For this review, use the dimensioned drawing (mm, ordinates from the lowest corner) and the shaded views. Coordinates: 2 decimals unless noted, no trailing zeros. Write each loop counter-clockwise with the first axis right and the second up, starting at its lowest first coordinate (ties: lowest second). Pieces come first, ordered by that corner, then holes.
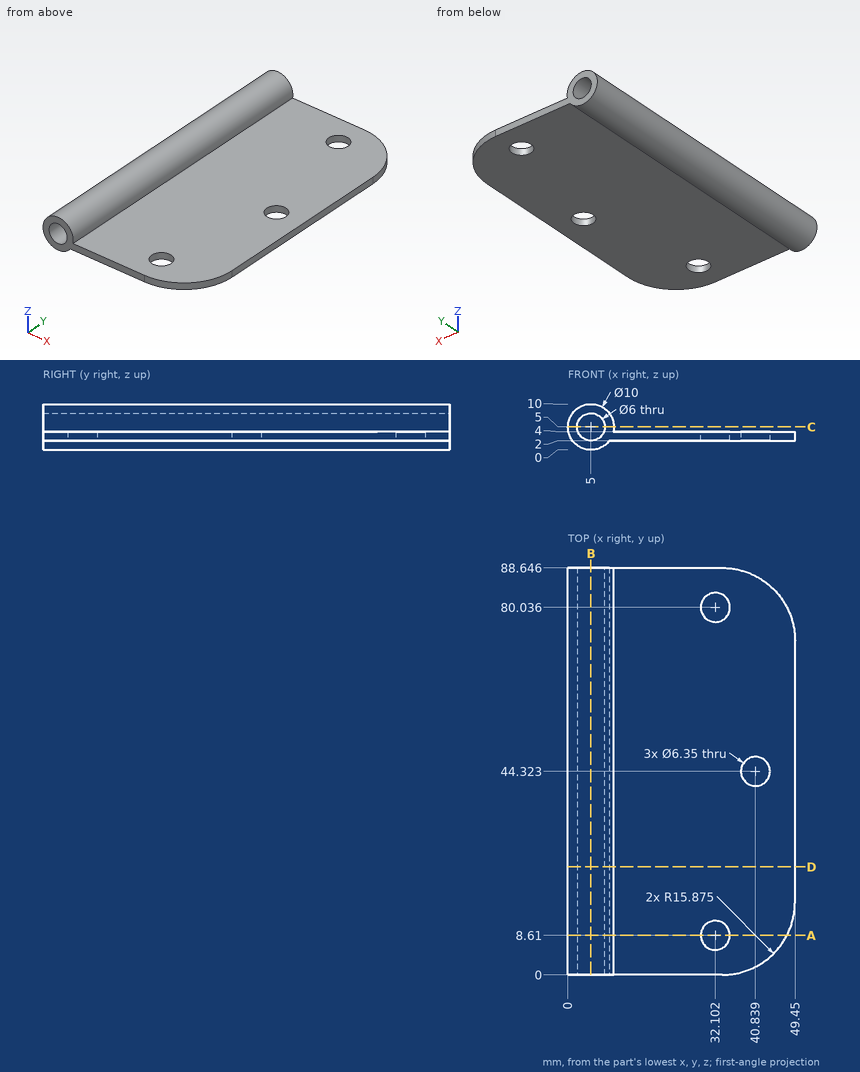
Item 1: Take a section at A-A, the plane y = 8.61. Write out the cut boundary in (x, z).
Solved:
outline: (9, 2) - (28.93, 2) - (28.93, 4) - (9.9, 4) arc R5 ccw (long way) to start; (35.28, 2) - (47.69, 2) - (47.69, 4) - (35.28, 4) - close; hole circle Ø6 at (5, 5)
Item 2: Take a section at D-D, the plane y = 23.5. Write out the cut boundary in (x, z).
Solved:
outline: (9, 2) - (49.45, 2) - (49.45, 4) - (9.9, 4) arc R5 ccw (long way) to start; hole circle Ø6 at (5, 5)
Item 3: For pin 1 (10 mm diameter, centred on x = 32.1, y = 80.04, fed in from +Z); pin 2 (5 mm diameter, centred on x = 17.5, y = 39, fed in from -Z); pin 3 (2 mm diameter, centred on x = 36, z = 4, fed in from -Y), all flat-tipped, find the tip position at first contact; note any pin that passes through.
Solved:
pin 1: stops at z = 4
pin 2: stops at z = 2
pin 3: stops at y = 0.06
Item 4: Take a section at C-C, the plane z = 5. Write out the cut boundary in (x, y).
Solved:
outline: (0, 0) - (2, 0) - (2, 88.65) - (0, 88.65) - close; (8, 0) - (10, 0) - (10, 88.65) - (8, 88.65) - close
Item 5: To check wall thickness, follow line 1 along Y through (x, z) = (34.5, 3.5) (1 decimal); line 2 along Z through (x, y) = (5, 28.5); line 3 along Z through (x, y) = (29.5, 24). State the ranges of each line that lie inside material, in increasing order.
Solved:
line 1: y = 0 to 6.5, 10.7 to 78, 82.1 to 88.6
line 2: z = 0 to 2, 8 to 10
line 3: z = 2 to 4
Item 6: Take a section at B-B, the plane x = 5. Write out the cut boundary in (y, z).
Solved:
outline: (0, 0) - (88.65, 0) - (88.65, 2) - (0, 2) - close; (0, 8) - (88.65, 8) - (88.65, 10) - (0, 10) - close
